Part model, mm, in its own coordinate system. A direction names the side the tool comes from. Coordinates: 2 decimals unless noted, no trailing zeros. Loops run counter-clockwise (first coordinate to the right, second up) from the corner with the lowest first, then second, coordinate; pieces in that order, holes last. Notation, with made-up numbers: M -24,15.5 L 17,15.5 A20 cw 17,20.5 Z; hole C 57.5,-22 d8. An arc over 180 degrees is marked long. Use CSV: the item, a comma, the result in double quotes. Start each with the question number.
from build123d import *

# Parameters (mm, degrees)
F0_W     = 1701.8
F0_H     = 1143
F1_DEPTH = 1422.4
F2_R     = 80.01
F3_DEPTH = 160.02
F5_DEPTH = 38.1
F6_W     = 83.82
F6_H     = 736.6
F7_DEPTH = 25.4
F9_DEPTH = 965.2


with BuildPart() as f1:
    # F0 (on Top) → F1 (new body)
    with BuildSketch(Plane.XY):
        with Locations((-6.391168, -71.989974)):
            Rectangle(F0_W, F0_H)
    extrude(amount=F1_DEPTH)

    # F2 (on face) → F3 (cut)
    with BuildSketch(Plane(origin=(0, 499.510026, 0), x_dir=(-1, 0, 0), z_dir=(0, 1, 0))):
        with Locations((-553.678832, 930.91)):
            Circle(F2_R)
    extrude(amount=-F3_DEPTH, mode=Mode.SUBTRACT)

    # F4 (on face) → F5 (cut)
    with BuildSketch(Plane.XY.offset(1422.4)):
        Polygon((-857.291168, -643.489974), (-735.371168, -643.489974), (-6.391168, -172.348559), (722.588832, -643.489974), (844.508832, -643.489974), (844.508832, -521.569974), (148.890026, -71.989974), (844.508832, 377.590026), (844.508832, 499.510026), (722.588832, 499.510026), (-6.391168, 28.368612), (-735.371168, 499.510026), (-857.291168, 499.510026), (-857.291168, 377.590026), (-161.672362, -71.989974), (-857.291168, -521.569974), align=None)
    extrude(amount=-F5_DEPTH, mode=Mode.SUBTRACT)

    # F6 (on face) → F7 (cut)
    with BuildSketch(Plane.YZ.offset(844.508832)):
        with Locations((140.100026, 368.3)):
            Rectangle(F6_W, F6_H)
    extrude(amount=-F7_DEPTH, mode=Mode.SUBTRACT)

    # F8 (on face) → F9 (cut)
    with BuildSketch(Plane.YZ.offset(844.508832)):
        with BuildLine():
            Line((14.370026, 0), (14.370026, 38.1))
            ThreePointArc((14.370026, 38.1), (-226.929974, 458.349814), (-468.229974, 38.1))
            Line((-468.229974, 38.1), (-468.229974, 0))
            Line((-468.229974, 0), (14.370026, 0))
        make_face()
    extrude(amount=-F9_DEPTH, mode=Mode.SUBTRACT)


solid = f1.part
1. Slice it at A-A, the plane y = 399. List the corners of the cut face in (x, z).
2. Tool access for faces 1 (the face through (-514.351, 155.947, 1403.617)), 2 (the face through (369, 14.37, 19)), 3 (the face through (368.67, -218.72, 458.23)), 4 (the face through (564.09, 420.62, 1010.24)): list every direction of +Z, -Z, +X, -X, +Y, -Y with a clear straight run to the whole face (end or side of a thin tool).
3. Slice it at B-B, the plane z = 118. List the corners of the cut face in (x, y), and give its area (3 significant figures).
4. Pin check, flat tips, straight feed: pin 1 (12.5 mm diameter, centred on x = 826.5, y = 131, fed in from -Z); pin 2 (12 mm diameter, centred on x = -481.5, y = -395, fed in from -Z). Stop position of each tip, or through.
5. Wall check: probe 1 along Z at (x, y) = (-465, 173.5); probe 2 along Y at (x, z) = (136, 169.5); probe 3 along Y at (x, z) = (763.5, 347.5). Give the ranges that are in metal, low to high.
6. Slice it at C-C, the plane y = -250. List the corners of the cut face in (x, z), and give its area (3 significant figures).
7. Two-plate mould, pull along Y, no slides. Class faces 5 (the face through (501.57, -299.93, 1403.62)), 6 (the face through (555, 339.49, 932)), 7 (the face through (-18, -643.49, 701)): pulls with the +Y half, pulls with the -Y half, needs draft (parallel to the pull), parting line crosses it, or undercut.
Found:
1,outline,"M -857.29,0 L 844.51,0 L 844.51,1384.3 L 567.07,1384.3 L 567.07,1422.4 L -579.86,1422.4 L -579.86,1384.3 L -857.29,1384.3 Z; hole C 553.68,930.91 d160.02"
2,face 1,"+Z"
2,face 2,"-Z, +X"
2,face 3,"+X"
2,face 4,"+Y"
3,outline,"M -857.29,-643.49 L 844.51,-643.49 L 844.51,-499.6 L -120.69,-499.6 L -120.69,45.74 L 844.51,45.74 L 844.51,98.19 L 819.11,98.19 L 819.11,182.01 L 844.51,182.01 L 844.51,499.51 L -857.29,499.51 Z"
3,area,"1,420,000 mm^2"
4,pin 1,"z = 736.6"
4,pin 2,"z = 0"
5,probe 1,"0 to 1384.3"
5,probe 2,"-643.49 to -506.17, 52.31 to 499.51"
5,probe 3,"-643.49 to -449.76, -4.1 to 499.51"
6,outline,"M -857.29,0 L -120.69,0 L -120.69,457.4 L 844.51,457.4 L 844.51,1422.4 L 424.32,1422.4 L 424.32,1384.3 L 113.76,1384.3 L 113.76,1422.4 L -126.54,1422.4 L -126.54,1384.3 L -437.1,1384.3 L -437.1,1422.4 L -857.29,1422.4 Z"
6,area,"1,960,000 mm^2"
7,face 5,"undercut"
7,face 6,"pulls with the +Y half"
7,face 7,"pulls with the -Y half"
